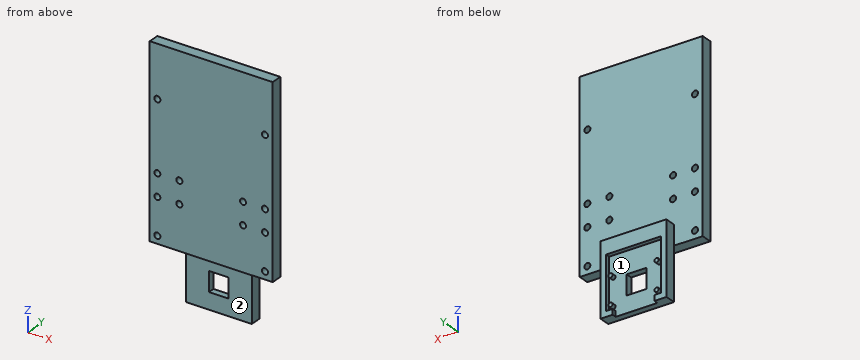
from build123d import *

# Parameters (mm, degrees)
SKETCH1_W           = 56
SKETCH1_H           = 85
BOSS_EXTRUDE1_DEPTH = 5
SKETCH2_R           = 1.375
CUT_EXTRUDE1_DEPTH  = 5
SKETCH3_R           = 1.375
CUT_EXTRUDE2_DEPTH  = 5
SKETCH5_W           = 30
SKETCH5_H           = 8.938360197
BOSS_EXTRUDE2_DEPTH = 5
SKETCH6_W           = 30
SKETCH6_H           = 5
BOSS_EXTRUDE3_DEPTH = 24
CUT_EXTRUDE3_DEPTH  = 2
SKETCH9_W           = 9
SKETCH9_H           = 9
CUT_EXTRUDE4_DEPTH  = 3
SKETCH10_R          = 0.95
BOSS_EXTRUDE4_DEPTH = 2


with BuildPart() as part:
    # Sketch1 → Boss-Extrude1 (new body)
    with BuildSketch(Plane(origin=(0, 0, 0), x_dir=(1, 0, 0), z_dir=(0, 1, 0))):
        with Locations((-25.952095808, 2.54491018)):
            Rectangle(SKETCH1_W, SKETCH1_H)
    extrude(amount=BOSS_EXTRUDE1_DEPTH)

    # Sketch2 → Cut-Extrude1 (cut)
    with BuildSketch(Plane(origin=(0, 0, 0), x_dir=(-1, 0, 0), z_dir=(0, -1, 0))):
        with Locations(Location((50.452095808, 41.54491018, 0), (0, 0, 90))):
            Circle(SKETCH2_R)
        with Locations(Location((1.452095808, 41.54491018, 0), (0, 0, 90))):
            Circle(SKETCH2_R)
        with Locations(Location((50.452095808, -16.45508982, 0), (0, 0, 90))):
            Circle(SKETCH2_R)
        with Locations(Location((1.452095808, -16.45508982, 0), (0, 0, 90))):
            Circle(SKETCH2_R)
    extrude(amount=-CUT_EXTRUDE1_DEPTH, mode=Mode.SUBTRACT)

    # Sketch3 → Cut-Extrude2 (cut)
    with BuildSketch(Plane(origin=(0, 0, 0), x_dir=(-1, 0, 0), z_dir=(0, -1, 0))):
        with Locations(Location((50.452095808, 25.04491018, 0), (0, 0, 90))):
            Circle(SKETCH3_R)
        with Locations(Location((50.452095808, 15.04491018, 0), (0, 0, 90))):
            Circle(SKETCH3_R)
        with Locations(Location((40.452095808, 15.04491018, 0), (0, 0, 90))):
            Circle(SKETCH3_R)
        with Locations(Location((40.452095808, 25.04491018, 0), (0, 0, 90))):
            Circle(SKETCH3_R)
        with Locations(Location((1.452095808, 25.04491018, 0), (0, 0, 90))):
            Circle(SKETCH3_R)
        with Locations(Location((11.452095808, 25.04491018, 0), (0, 0, 90))):
            Circle(SKETCH3_R)
        with Locations(Location((1.452095808, 15.04491018, 0), (0, 0, 90))):
            Circle(SKETCH3_R)
        with Locations(Location((11.452095808, 15.04491018, 0), (0, 0, 90))):
            Circle(SKETCH3_R)
    extrude(amount=-CUT_EXTRUDE2_DEPTH, mode=Mode.SUBTRACT)

    # Sketch5 → Boss-Extrude2 (add)
    with BuildSketch(Plane(origin=(0, 5, 0), x_dir=(1, 0, 0), z_dir=(0, 1, 0))):
        with Locations((-25.952095808, 40.575730081)):
            Rectangle(SKETCH5_W, SKETCH5_H)
    extrude(amount=BOSS_EXTRUDE2_DEPTH)

    # Sketch6 → Boss-Extrude3 (add)
    with BuildSketch(Plane(origin=(0, 0, -45.04491018), x_dir=(-1, 0, 0), z_dir=(0, 0, -1))):
        with Locations((25.952095808, 7.5)):
            Rectangle(SKETCH6_W, SKETCH6_H)
    extrude(amount=BOSS_EXTRUDE3_DEPTH)

    # Sketch8 → Cut-Extrude3 (cut)
    with BuildSketch(Plane(origin=(0, 10, 0), x_dir=(1, 0, 0), z_dir=(0, 1, 0))):
        Polygon((-38.452095808, 66.54491018), (-35.452095808, 66.54491018), (-35.452095808, 69.04491018), (-16.452095808, 69.04491018), (-16.452095808, 66.54491018), (-13.452095808, 66.54491018), (-13.452095808, 42.54491018), (-38.452095808, 42.54491018), align=None)
    extrude(amount=-CUT_EXTRUDE3_DEPTH, mode=Mode.SUBTRACT)

    # Sketch9 → Cut-Extrude4 (cut)
    with BuildSketch(Plane(origin=(0, 8, 0), x_dir=(1, 0, 0), z_dir=(0, 1, 0))):
        with Locations((-25.952095808, 57.04491018)):
            Rectangle(SKETCH9_W, SKETCH9_H)
    extrude(amount=-CUT_EXTRUDE4_DEPTH, mode=Mode.SUBTRACT)

    # Sketch10 → Boss-Extrude4 (add)
    with BuildSketch(Plane(origin=(0, 8, 0), x_dir=(1, 0, 0), z_dir=(0, 1, 0))):
        with Locations(Location((-36.452095808, 64.54491018, 0), (0, 0, 270))):
            Circle(SKETCH10_R)
        with Locations(Location((-15.452095808, 64.54491018, 0), (0, 0, 270))):
            Circle(SKETCH10_R)
        with Locations(Location((-15.452095808, 52.04491018, 0), (0, 0, 270))):
            Circle(SKETCH10_R)
        with Locations(Location((-36.452095808, 52.04491018, 0), (0, 0, 270))):
            Circle(SKETCH10_R)
    extrude(amount=BOSS_EXTRUDE4_DEPTH)


solid = part.part
Part model, mm, in its own coordinate system. Face numbers are marked on the shaded views. Give positions to 0.01 mm unless a question says otherwise; leave off trailing zeros. Loops run counter-clockwise (first coordinate to the right, second up) from the corner with the lowest first, then second, coordinate; pieces in that order, holes last.
(1) Band-saw the part on D-D (z = 12.5). Write the cut outline in (x, y).
Return value:
outline: (-53.95, 0) - (2.05, 0) - (2.05, 5) - (-53.95, 5) - close
(2) Pin check, flat tips, straight feed: pin 1 (4 mm diameter, centred on x = -12.5, z = -7.5, fed in from +Y); pin 2 (1.5 mm diameter, centred on y = 7, z = -56.5, fed in from -X); pin 3 (0.9 mm diameter, centred on y = 7, z = -56.5, fed in from +X). Stop position of each tip, or through.
Return value:
pin 1: stops at y = 5
pin 2: stops at x = -40.95
pin 3: stops at x = -10.95
(3) Band-saw the part on B-B (y = 7). Write the cut outline in (x, z).
Return value:
outline: (-40.95, -69.04) - (-10.95, -69.04) - (-10.95, -36.11) - (-40.95, -36.11) - close; hole (-30.45, -61.54) - (-21.45, -61.54) - (-21.45, -52.54) - (-30.45, -52.54) - close
(4) Pull direction X, two halves, no side cores. Call the marked faces 1 and 2: pulls with the +X half, pulls with the -X half, needs draft (parallel to the pull), parting line crosses it, or undercut.
Return value:
face 1: undercut
face 2: needs draft
(5) Drill centre lines: line 1 along Z through (x, y) = (-1, 1.25); line 2 along Z through (x, y) = (-33, 4.25); line 3 along Z through (x, y) = (-16, 7.5). Where is each one in solid material? Low to high.
Return value:
line 1: z = -45.04 to -42.84, -40.25 to -26.34, -23.75 to -16.34, -13.75 to 15.16, 17.75 to 39.96
line 2: z = -45.04 to 39.96
line 3: z = -69.04 to -36.11
(6) Band-saw the part on A-A (x = -22.5). Write the cut outline in (y, z), and give its area (3 significant figures).
Return value:
outline: (0, -45.04) - (5, -45.04) - (5, -52.54) - (8, -52.54) - (8, -42.54) - (10, -42.54) - (10, -36.11) - (5, -36.11) - (5, 39.96) - (0, 39.96) - close; (5, -69.04) - (8, -69.04) - (8, -61.54) - (5, -61.54) - close
area: 510 mm2
(7) Band-saw the part on C-C (z = -58). Write the cut outline in (x, y).
Return value:
outline: (-40.95, 5) - (-30.45, 5) - (-30.45, 8) - (-38.45, 8) - (-38.45, 10) - (-40.95, 10) - close; (-21.45, 5) - (-10.95, 5) - (-10.95, 10) - (-13.45, 10) - (-13.45, 8) - (-21.45, 8) - close
